Design review of the part built by this model. Coordinates are the model's own, in mm. A direction names the side the tool comes from. Give positions to 0.01 mm unless a question says otherwise; leave off trailing zeros. Order: outer loops, then holes, each group sorted by start corner. A loop starts at its lowest first (then second) coordinate and runs counter-clockwise, first axis right, second up.
```python
from build123d import *

# Parameters (mm, degrees)
F0_W      = 107.95
F0_H      = 90.4875
F1_DEPTH  = 7.14375
F2_W      = 101.6
F2_H      = 81.75625
F3_DEPTH  = 3.96875
F4_W      = 101.6
F4_H      = 4.7625
F4_H_2    = 5.55625
F5_DEPTH  = 2.38125
F6_W      = 11.90625
F6_H      = 2.38125
F7_DEPTH  = 25.4
F8_R      = 0.79375
F9_DEPTH  = 25.4
F10_R     = 3.175
F11_R     = 1.5875
F11_R_2   = 0.79375
F12_DEPTH = 1.5875


with BuildPart() as f1:
    # F0 (on Top) → F1 (new body)
    with BuildSketch(Plane.XY):
        Rectangle(F0_W, F0_H)
    extrude(amount=F1_DEPTH)

    # F2 (on face) → F3 (cut)
    with BuildSketch(Plane.XY.offset(7.14375)):
        with Locations((0, -1.190625)):
            Rectangle(F2_W, F2_H)
    extrude(amount=-F3_DEPTH, mode=Mode.SUBTRACT)

    # F4 (on face) → F5 (join)
    with BuildSketch(Plane.XY.offset(3.175)):
        with Locations((0, 37.30625)):
            Rectangle(F4_W, F4_H)
        with Locations((0, -39.290625)):
            Rectangle(F4_W, F4_H_2)
    extrude(amount=F5_DEPTH)

    # F6 (on face) → F7 (cut)
    with BuildSketch(Plane.XZ.offset(45.24375)):
        with Locations((-40.084375, 5.953125)):
            Rectangle(F6_W, F6_H)
    extrude(amount=-F7_DEPTH, mode=Mode.SUBTRACT)

    # F8 (on face) → F9 (cut)
    with BuildSketch(Plane.XY.offset(5.55625)):
        with Locations((48.815625, 36.909375)):
            Circle(F8_R)
        with Locations((48.815625, -39.290625)):
            Circle(F8_R)
        with Locations((-48.41875, 36.909375)):
            Circle(F8_R)
    extrude(amount=-F9_DEPTH, mode=Mode.SUBTRACT)

    # F10
    f10_edges = [f1.edges().sort_by_distance(p)[0] for p in [
        (53.975, -45.24375, 3.571875),
        (53.975, 45.24375, 3.571875),
        (-53.975, 45.24375, 3.571875),
        (-53.975, -45.24375, 3.571875),
        (0, -45.24375, 0),
        (-53.975, 0, 0),
        (0, 45.24375, 0),
        (53.975, 0, 0),
    ]]
    fillet(f10_edges, radius=F10_R)

    # F11 (on face) → F12 (cut)
    with BuildSketch(Plane(origin=(0, 0, 0), x_dir=(1, 0, 0), z_dir=(0, 0, -1))):
        with Locations((-48.41875, -36.909375)):
            Circle(F11_R)
        with Locations((-48.41875, -36.909375)):
            Circle(F11_R_2, mode=Mode.SUBTRACT)
        with Locations((48.815625, -36.909375)):
            Circle(F11_R)
        with Locations((48.815625, -36.909375)):
            Circle(F11_R_2, mode=Mode.SUBTRACT)
        with Locations((48.815625, 39.290625)):
            Circle(F11_R)
        with Locations((48.815625, 39.290625)):
            Circle(F11_R_2, mode=Mode.SUBTRACT)
    extrude(amount=-F12_DEPTH, mode=Mode.SUBTRACT)


solid = f1.part
```
1. Machinability: for faces 4 (the face through (-46.038, -42, 5)), 5 (the face through (48.47, -37.74, 0.78)), 6 (the face through (-1, 34.925, 4)), which of the approach directions +Z, -Z, +X, -X, +Y, -Y give a long, thin tool a straight path to every point of the face, cutting with its end or side? Answer none if there is none.
Recorded:
face 4: +Z, -Y
face 5: -Z
face 6: +Z
2. Take a section at A-A (y = 13). State the section outline as (x, z) points (3 decimals).
Recorded:
outline: (-53.975, 3.175) arc R3.175 ccw to (-50.8, 0) - (50.8, 0) arc R3.175 ccw to (53.975, 3.175) - (53.975, 7.144) - (50.8, 7.144) - (50.8, 3.175) - (-50.8, 3.175) - (-50.8, 7.144) - (-53.975, 7.144) - close
3. For pin 1 (3 mm diameter, centred on x = 48.82, y = -39.29, fed in from -Z); pin 2 (1.6 mm diameter, centred on x = 48, y = 36.5, fed in from -Z); pin 3 (7 mm diameter, centred on x = -38.5, y = -42, fed in from +Z); pin 4 (1.9 mm diameter, centred on x = 48.82, y = 36.91, fed in from +Z), all flat-tipped, find the tip position at first contact; note any pin that passes through.
Recorded:
pin 1: stops at z = 1.59
pin 2: stops at z = 0
pin 3: stops at z = 4.76
pin 4: stops at z = 5.56
4. Draft analysis for pull direction X (two halves, no side actions). For faces 1 (the face through (48.47, 38.46, 0.78)), 2 (the face through (-53.07, 0.589, 0.955)), 3 (the face through (0.711, 44.338, 0.955)), state which applies: pulls with the +X half, pulls with the -X half, needs draft (parallel to the pull), parting line crosses it, or undercut.
Recorded:
face 1: undercut
face 2: pulls with the -X half
face 3: needs draft
5. For line 1 along Y through (x, z) = (26, 3.75) (1 decimal); line 2 along X through (y, z) = (29.5, 6.5) (3 decimals); line 3 along Y through (x, z) = (2, 5.75), list the stretches that pass through material, from the lowest coordinate up.
Recorded:
line 1: y = -45.2 to -36.5, 34.9 to 45.2
line 2: x = -53.975 to -50.8, 50.8 to 53.975
line 3: y = -45.24 to -42.07, 39.69 to 45.24
